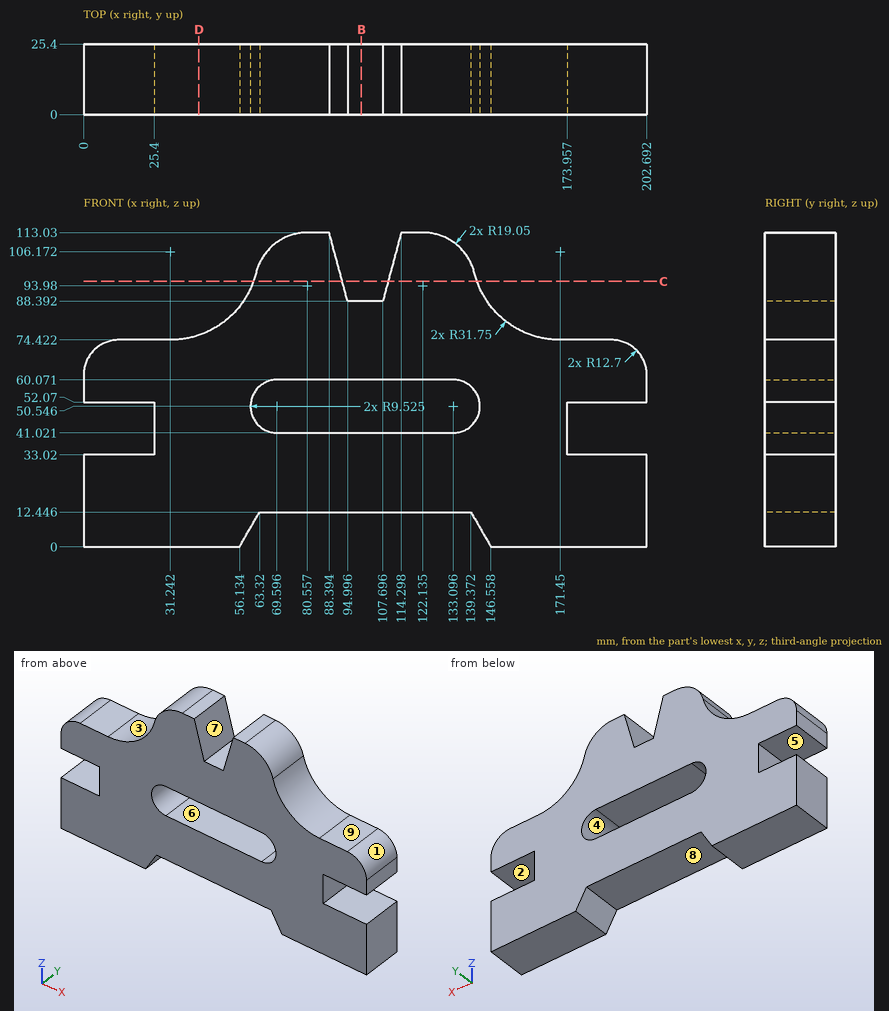
Geometry check sheet. Reference: drawing and pictorial views, mm from the part's lowest x, y, z. A direction names the side the tool comes from. Give positions to 0.01 mm unless a question says otherwise; leave off trailing zeros. Order: outer loops, then holes, each group sorted by start corner. A loop starts at its lowest first (then second) coordinate and runs counter-clockwise, first axis right, second up. Notation, with made-up numbers: M 13,73.5 L 56,73.5 A18 cw 56,91.5 Z; hole C 77,-9 d11. An arc over 180 degrees is marked long. Answer as a JSON object with one key per item and string values. Group by question number.
1) Mould release check, pull along X, two halves, no side actions. Record for the marked faces 1, 2, 3 and 4: released by +X, released by -X, zero draft, split by the parting line, or undercut.
2) Depth check by flat-ended pin: pin 1 Ø3 at (x, y) = (79.5, 18.5) entering from -Z; pin 2 Ø9.5 at (y, z) = (16.5, 46) entering from +X; pin 3 Ø4 at (y, z) = (8.5, 88.5) entering from +X. Enter the tip coordinate at first touch or a pass-through.
3) Scan lines: line 1 along Z through (x, y) = (181, 16); line 2 along Z through (x, y) = (115, 8); line 3 along X through (y, z) = (13, 86.5) (1 decimal). Record each from-to range of solid material in increasing order. Write a range as [from, to].
4) Cross-section at D-D (x = 41.5). Enter the section's corners in (y, z) (1 decimal), then the cut area to 3 significant figures.
5) Cross-section at C-C (z = 95.5). Enter the section's corners in (x, y) (1 decimal).
6) Access from +Z, -Z, +X, -X, +Y, -Y to the whole of each face (thin tool, end or side, straight path). Record for the marked faces 5, 6, 7, 8 and 9.
7) Cross-section at B-B (x = 100). Enter the section's corners in (y, z), then the cut area to 4 significant figures.
Result sheet:
{
 "1": {"face 1": "released by +X", "face 2": "zero draft", "face 3": "released by -X", "face 4": "undercut"},
 "2": {"pin 1": "stops at z = 12.45", "pin 2": "stops at x = 173.96", "pin 3": "stops at x = 146.53"},
 "3": {"line 1": "z = [0, 33.02], [52.07, 74.42]", "line 2": "z = [12.45, 41.02], [60.07, 113.03]", "line 3": "x = [56.2, 146.5]"},
 "4": {"outline": "M 0,0 L 25.4,0 L 25.4,76.1 L 0,76.1 Z", "area": "1,930 mm2"},
 "5": {"outline": "M 61.1,0 L 93.1,0 L 93.1,25.4 L 61.1,25.4 Z; M 109.6,0 L 141.5,0 L 141.5,25.4 L 109.6,25.4 Z"},
 "6": {"face 5": "-X, +Y, -Y", "face 6": "+Y, -Y", "face 7": "+Z, +Y, -Y", "face 8": "-Z, +Y, -Y", "face 9": "+Z, +X, +Y, -Y"},
 "7": {"outline": "M 0,12.45 L 25.4,12.45 L 25.4,41.02 L 0,41.02 Z; M 0,60.07 L 25.4,60.07 L 25.4,88.39 L 0,88.39 Z", "area": "1,445 mm2"}
}
